```python
from build123d import *

# Parameters (mm, degrees)
F0_R     = 3.175
F1_DEPTH = 3.175


with BuildPart() as f1:
    # F0 (on Top) → F1 (new body)
    with BuildSketch(Plane.XY):
        with BuildLine():
            Line((0, 38.1), (0, 0))
            ThreePointArc((0, 0), (3.772278, -24.826826), (7.544557, 0))
            Line((7.544557, 0), (11.865513, 9.914308))
            Line((11.865513, 9.914308), (7.544557, 12.825744))
            Line((7.544557, 12.825744), (11.865513, 19.238615))
            Line((11.865513, 19.238615), (7.544557, 26.40594))
            Line((7.544557, 26.40594), (11.865513, 38.1))
            Line((11.865513, 38.1), (4.149509, 43.758412))
            Line((4.149509, 43.758412), (0, 38.1))
        make_face()
        with Locations((3.772278, -12.126826)):
            Circle(F0_R, mode=Mode.SUBTRACT)
    extrude(amount=F1_DEPTH)


solid = f1.part
```
Geometry: final body of the model. Coordinates: model frame, mm. A direction names the side the tool comes from. Give positions to 0.01 mm unless a question says otherwise; leave off trailing zeros. Order: outer loops, then holes, each group sorted by start corner. A loop starts at its lowest first (then second) coordinate and runs counter-clockwise, first axis right, second up. Notation, with made-up numbers: M 9,1 L 24,1 A8 cw 24,10 Z; hole C -12,27.5 d7. An arc over 180 degrees is marked long. Answer as CSV lines item,"result". Start each with the question number.
1) Mould query, pull axis Y, two halves, no side actions, for faces 1 (the flat face through (9.735, 22.772, 1.565)), 2 (the flat face through (8.06, 40.89, 1.57)), 3 (the flat face through (4, 2, 0)). Classes: +Y half, -Y half, draft (parallel to the pull), parting line (faces both ways), or undercut.
2) First-contact query: P1, Ø1.5, axis at y = 4.5, z = 2, coming from the +X side; P2, Ø1, axis at x = 5, y = -11, coming from the +Z side; P3, Ø1.5, axis at y = 11, z = 0.5, coming from the +X side. Flat tips, straight axial feed; report the tip coordinate or a pass-through.
3) Line query: line 1 (Y direction, x = 4, z = 1.4); line 2 (Y direction, x = 5.25, z = 2.8); line 3 (X direction, y = -13, z = 0.4). Output: solid intervals per line, ascending. Write a range as from..to.
4) Cut plane D-D (y = -6). Output: boundary loops of the cut face in (x, z) (3 decimals), then the cut area to 3 significant figures.
5) Set-up query: faces 4 (the flat face through (0, 19, 2)), 5 (the flat face through (9.675, 32.171, 1.565)), 6 (the cylindrical face through (1.432, -9.981, 1.565)). Return all of +Z, -Z, +X, -X, +Y, -Y with unobstructed straight access to the full face (end or side cutting, diameter ignored); none if empty.
6) Cut plane C-C (x = 9.75). Output: boundary loops of the cut face in (y, z) (3 decimals), then the cut area to 3 significant figures.
7) Cut plane A-A (x = 2). Output: boundary loops of the cut face in (y, z) (1 decimal).
Findings below:
1,face 1,"undercut"
1,face 2,"+Y half"
1,face 3,"draft"
2,P1,"stops at x = 9.83"
2,P2,"passes through"
2,P3,"stops at x = 11.37"
3,line 1,"y = -24.82..-15.29, -8.96..43.55"
3,line 2,"y = -24.74..-14.94, -9.32..42.95"
3,line 3,"x = -8.9..0.72, 6.82..16.44"
4,outline,"M -7.352,0 L 14.897,0 L 14.897,3.175 L -7.352,3.175 Z"
4,area,"70.6 mm²"
5,face 4,"+Z, -Z, -X, +Y"
5,face 5,"+Z, -Z, +X"
5,face 6,"+Z, -Z"
6,outline,"M -23.332,0 L -0.922,0 L -0.922,3.175 L -23.332,3.175 Z; M 5.06,0 L 11.34,0 L 11.34,3.175 L 5.06,3.175 Z; M 16.099,0 L 22.748,0 L 22.748,3.175 L 16.099,3.175 Z; M 32.375,0 L 39.651,0 L 39.651,3.175 L 32.375,3.175 Z"
6,area,"135 mm²"
7,outline,"M -24.7,0 L -14.8,0 L -14.8,3.2 L -24.7,3.2 Z; M -9.5,0 L 40.8,0 L 40.8,3.2 L -9.5,3.2 Z"
